```python
from build123d import *

# Parameters (mm, degrees)
F1_DEPTH = 3
F4_DEPTH = 3
F6_W     = 3
F6_H     = 50
F7_DEPTH = 305
F8_W     = 2036.6446971893
F8_H     = 607.4184775352
F9_DEPTH = 2


with BuildPart() as f1:
    # F0 (on Front) → F1 (new body)
    with BuildSketch(Plane.XZ):
        Polygon((1000, 0), (0, 0), (-1064.7249259854, -220.0647401601), (-1064.7249259854, -400.0647401601), (1000, -71.1974114174), align=None)
    extrude(amount=F1_DEPTH)

    # F6 (on offset) → F7, piece 2 (join, symmetric)
    with BuildSketch(Plane.XZ.offset(303)):
        with Locations((167.9982813472, 25)):
            Rectangle(F6_W, F6_H)
        with Locations((397.9982813472, 25)):
            Rectangle(F6_W, F6_H)
        with Locations((627.9982813472, 25)):
            Rectangle(F6_W, F6_H)
        with Locations((857.9982813472, 25)):
            Rectangle(F6_W, F6_H)
    extrude(amount=F7_DEPTH, both=True)



with BuildPart() as f4:
    # F3 (on offset) → F4 (new body)
    with BuildSketch(Plane.XZ.offset(603)):
        Polygon((994.6181178093, -157.9961776733), (0, 0), (-1063.7367963791, 0), (-1063.7367963791, -74.729397893), (0, -227.9402762651), (994.6181178093, -344.5137739182), align=None)
    extrude(amount=F4_DEPTH)

    # F6 (on offset) → F7 (join, symmetric)
    with BuildSketch(Plane.XZ.offset(303)):
        with Locations((-982.0017186528, 25)):
            Rectangle(F6_W, F6_H)
        with Locations((-752.0017186528, 25)):
            Rectangle(F6_W, F6_H)
        with Locations((-522.0017186528, 25)):
            Rectangle(F6_W, F6_H)
        with Locations((-292.0017186528, 25)):
            Rectangle(F6_W, F6_H)
        with Locations((-62.0017186528, 25)):
            Rectangle(F6_W, F6_H)
    extrude(amount=F7_DEPTH, both=True)


with BuildPart() as f1_1:
    add(f1.part)

    add(f4.part)  # F9 merges F4
    # F8 (on face) → F9 (join)
    with BuildSketch(Plane.XY.offset(50)):
        with Locations((-30.8758020401, -303.7092387676)):
            Rectangle(F8_W, F8_H)
    extrude(amount=F9_DEPTH)


solid = f1_1.part
```
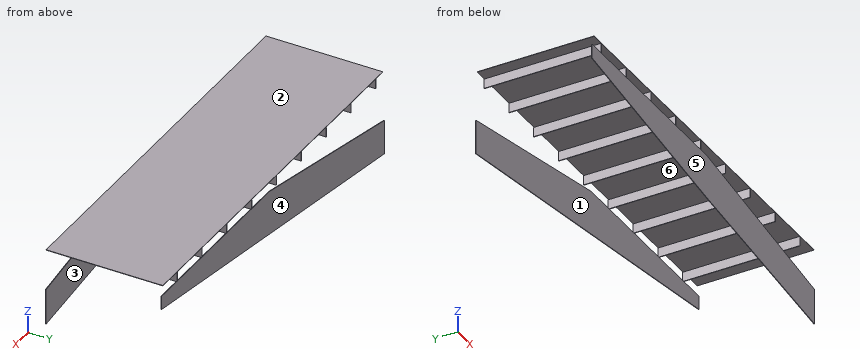
CAD build for the part. Positions are in the model's coordinates, mm. Face numbers are marked on the shaded views. A direction names the side the tool comes from. Round coordinates to 2 decimals unless told otherwise and drop trailing zeros. Order: outer loops, then holes, each group sorted by start corner. A loop starts at its lowest first (then second) coordinate and runs counter-clockwise, first axis right, second up.
Item 1: Saw through at B-B on z = -27.5. Write the cut outline in (x, y).
Item 2: Probe line 1 along Y through (x, z) = (302.5, -173); line 2 along Z through (x, y) = (593, -494); line 3 along Y through (x, z) = (787.5, -18). List the from-to ranges inside material, lowest first.
Item 3: Mould opens along Y. For the marked faces 3, 4, 5 and 6 say: pulls with the +Y half, pulls with the -Y half, needs draft (parallel to the pull), parting line crosses it, or undercut.
Item 4: Saw through at D-D on z = -136. Write the cut outline in (x, y), then the cut area to 3 significant figures.
Item 5: Saw through at C-C on x = -443.5. Write the cut outline in (y, z), then the cut area to 3 significant figures.
Item 6: Pin check, flat tips, straight feed: pin 1 (0.9 mm diameter, centred on x = -752, y = -214, fed in from -Z); pin 2 (15 mm diameter, centred on y = -376, z = 20.5, fed in from +X); pin 3 (3.5 mm diameter, centred on y = -604, z = -37.5, fed in from -X). Stop position of each tip, or through.
Item 7: Saw through at A-A on x = 666.5. Write the cut outline in (y, z), then the cut area to 3 significant figures.
Item 8: Tool access for the marked faces 1 and 2: list every direction of +Z, -Z, +X, -X, +Y, -Y with a clear straight run to the whole face (end or side of a thin tool).
Reported:
1. outline: (-1063.74, -606) - (173.12, -606) - (173.12, -603) - (-1063.74, -603) - close; (-133.05, -3) - (1000, -3) - (1000, 0) - (-133.05, 0) - close
2. line 1: y = -606 to -603, -3 to 0
2. line 2: z = 50 to 52
2. line 3: y = -3 to 0
3. face 3: undercut
3. face 4: pulls with the +Y half
3. face 5: pulls with the -Y half
3. face 6: needs draft
4. outline: (-658, -3) - (593.15, -3) - (593.15, 0) - (-658, 0) - close; (-638.34, -606) - (856.15, -606) - (856.15, -603) - (-638.34, -603) - close
4. area: 8,240 mm2
5. outline: (-607.42, 50) - (0, 50) - (0, 52) - (-607.42, 52) - close; (-606, -164.06) - (-603, -164.06) - (-603, 0) - (-606, 0) - close; (-3, -301.12) - (0, -301.12) - (0, -91.67) - (-3, -91.67) - close
5. area: 2,340 mm2
6. pin 1: stops at z = 0
6. pin 2: stops at x = 859.5
6. pin 3: stops at x = -1063.74
7. outline: (-607.42, 50) - (0, 50) - (0, 52) - (-607.42, 52) - close; (-606, -306.06) - (-603, -306.06) - (-603, -105.87) - (-606, -105.87) - close; (-3, -124.32) - (0, -124.32) - (0, 0) - (-3, 0) - close
7. area: 2,190 mm2
8. face 1: -Z, +X, -X
8. face 2: +Z, +X, -X, +Y, -Y
